Could you check a few things on this model? Use its own coordinates, in mm. A direction names the side the tool comes from. Coordinates: 2 decimals unless noted, no trailing zeros. Loops run counter-clockwise (first coordinate to the right, second up) from the corner with the lowest first, then second, coordinate; pieces in that order, holes last.
1) Imagine slicing it at C-C on x = 69.5. Please give me the cut outline in (y, z), plus the area to 3 significant figures.
2) Thinking about a two-plate mould opening in Y: for faces 1 (the face through (405, -395, -10)), 2 (the face through (287, -287, 0)), 3 (the face through (0, -346, -10)), 4 (the face through (354, 0, -10)), which applies, released by +Y, released by -Y, zero draft, split by the parting line, or undercut?
3) If I drill on line 1 along Z through (x, y) = (154, -543); line 2 along Y through (x, z) = (252, -23); line 3 along X through (y, z) = (-646, -2), over which ranges is the centre line in solid material (lowest first)?
4) For faces 5 (the face through (247, -247, 5)), 6 (the face through (5, -348, -15)), 7 (the face through (391.614, -401.315, -14.79)), 8 (the face through (19.3, -50, 0.5)), which set-ups out of +Z, -Z, +X, -X, +Y, -Y let a thin tool reach every point of the face, with its end or its side?
5) Imagine slicing it at A-A on z = -8.5. Please give me the cut outline in (x, y).
6) Will these pins go through, and if not, where does the flat tip stop? P1, Ø24, axis at y = -436.5, z = -12, coming from the +X side; P2, Ø10, axis at x = 372.5, y = -321.5, coming from the +Z side; P3, Ø2, axis at y = -639.5, z = -10, coming from the +X side.
7) Imagine slicing it at B-B on y = -218.5. Please give me the cut outline in (x, z), plus the area to 3 significant figures.
```python
from build123d import *

# Parameters (mm, degrees)
F1_DEPTH  = 10
F2_R      = 5
F3_R      = 200
F4_DEPTH  = 5
F5_W      = 5
F5_H      = 690
F5_W_2    = 690
F5_H_2    = 5
F6_DEPTH  = 30
F7_W      = 50
F7_H      = 50
F8_DEPTH  = 40.001
F10_DEPTH = 40.001


with BuildPart() as f1:
    # F0 (on Top) → F1 (new body)
    with BuildSketch(Plane.XY):
        Polygon((750, 0), (0, 0), (0, -750), (50, -750), (750, -50), align=None)
    extrude(amount=F1_DEPTH)

    # F2
    f2_edges = [f1.edges().sort_by_distance(p)[0] for p in [
        (0, -750, 5),
        (750, 0, 5),
        (0, 0, 5),
    ]]
    fillet(f2_edges, radius=F2_R)

    # F3 (on face) → F4 (cut)
    with BuildSketch(Plane.XY.offset(10)):
        with Locations((250, -250)):
            Circle(F3_R)
    extrude(amount=-F4_DEPTH, mode=Mode.SUBTRACT)

    # F5 (on face) → F6 (join)
    with BuildSketch(Plane(origin=(0, 0, 0), x_dir=(1, 0, 0), z_dir=(0, 0, -1))):
        with Locations((2.5, 375)):
            Rectangle(F5_W, F5_H)
        with Locations((375, 2.5)):
            Rectangle(F5_W_2, F5_H_2)
        Polygon((750, 50), (50, 750), (46.4644660941, 746.4644660941), (746.4644660941, 46.4644660941), align=None)
    extrude(amount=F6_DEPTH)

    # F7 (on face) → F8 (cut, through all)
    with BuildSketch(Plane.XY.offset(10)):
        with Locations((25, -25)):
            Rectangle(F7_W, F7_H)
        with Locations((725, -25)):
            Rectangle(F7_W, F7_H)
        with Locations((25, -725)):
            Rectangle(F7_W, F7_H)
    extrude(amount=-F8_DEPTH, mode=Mode.SUBTRACT)

    # F9 (on face) → F10 (cut, through all)
    with BuildSketch(Plane.XY.offset(10)):
        Polygon((650, 0), (700, -50), (700, 0), align=None)
        Polygon((0, -650), (0, -700), (50, -700), align=None)
    extrude(amount=-F10_DEPTH, mode=Mode.SUBTRACT)


solid = f1.part
```
Filled in:
1. outline: (-730.5, -30) - (-723.43, -30) - (-723.43, 0) - (-5, 0) - (-5, -30) - (0, -30) - (0, 10) - (-163.86, 10) - (-163.86, 5) - (-336.14, 5) - (-336.14, 10) - (-730.5, 10) - close
1. area: 6,810 mm2
2. face 1: released by -Y
2. face 2: undercut
2. face 3: zero draft
2. face 4: released by +Y
3. line 1: z = 0 to 10
3. line 2: y = -548 to -540.93, -5 to 0
3. line 3: x = 0 to 5, 146.93 to 154
4. face 5: +Z
4. face 6: -Z, +Y, -Y
4. face 7: -Z
4. face 8: +Z, -Z, -X, +Y
5. outline: (0, -650) - (5, -655) - (5, -50) - (0, -50) - close; (50, -750) - (750, -50) - (742.93, -50) - (50, -742.93) - close; (50, -5) - (655, -5) - (650, 0) - (50, 0) - close
6. P1: stops at x = 375.5
6. P2: stops at z = 5
6. P3: stops at x = 161.5
7. outline: (0, -30) - (5, -30) - (5, 0) - (574.43, 0) - (574.43, -30) - (581.5, -30) - (581.5, 10) - (447.5, 10) - (447.5, 5) - (52.5, 5) - (52.5, 10) - (0, 10) - close
7. area: 4,200 mm2
